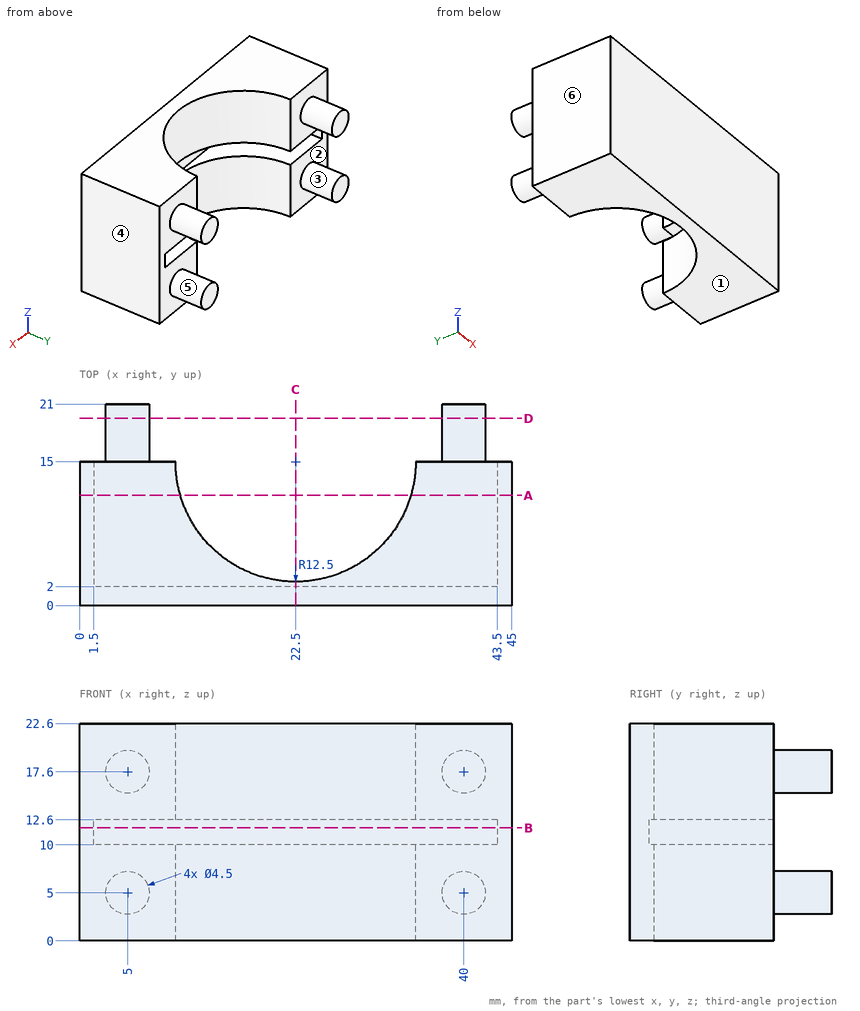
Job drawing, mm, ordinate dimensions from the low corner. One solid piece. A direction names the side the tool comes from. Round coordinates to 2 decimals unless told otherwise and drop trailing zeros. Write each loop counter-clockwise with the first axis right and the second up, starting at its lowest first coordinate (ties: lowest second). Pieces come first, ordered by that corner, then holes. Notation, with made-up numbers: (60, 65) -> (77, 65) arc R25 ccw to (77, 78) -> close; hole circle Ø5 at (31.5, 42.5). An arc over 180 degrees is marked (long way). Answer as a JSON object with one key per item and string values.
(1) Two-plate mould, pull along Z, no slides. Class the marked faces 1, 2, 3 and 4: +Z half, -Z half, draft (parallel to the pull), parting line (faces both ways), or undercut.
Reported:
{"face 1": "-Z half", "face 2": "undercut", "face 3": "undercut", "face 4": "draft"}
(2) Which spindle directions (+Z, -Z, +X, -X, +Y, -Y) get a long thin tool onto all of the face, cutting with end or side? Do the marked faces 5 and 6. Say none if no direction does.
Reported:
{"face 5": "+Y", "face 6": "+Z, -Z, -X, +Y, -Y"}
(3) Band-saw the part on A-A, the plane y = 11.5. List the corners of the cut face in (x, z), then the cut area to 3 significant figures.
Reported:
{"outline": "(0, 0) -> (10.5, 0) -> (10.5, 10) -> (1.5, 10) -> (1.5, 12.6) -> (10.5, 12.6) -> (10.5, 22.6) -> (0, 22.6) -> close; (34.5, 0) -> (45, 0) -> (45, 22.6) -> (34.5, 22.6) -> (34.5, 12.6) -> (43.5, 12.6) -> (43.5, 10) -> (34.5, 10) -> close", "area": "428 mm^2"}
(4) Band-saw the part on B-B, the plane z = 11.75. List the corners of the cut face in (x, y), then the cut area to 3 significant figures.
Reported:
{"outline": "(0, 0) -> (45, 0) -> (45, 15) -> (43.5, 15) -> (43.5, 2) -> (1.5, 2) -> (1.5, 15) -> (0, 15) -> close", "area": "129 mm^2"}
(5) Band-saw the part on D-D, the plane y = 19.5. List the corners of the cut face in (x, z), then the cut area to 3 significant figures.
Reported:
{"outline": "circle Ø4.5 at (5, 5); circle Ø4.5 at (5, 17.6); circle Ø4.5 at (40, 5); circle Ø4.5 at (40, 17.6)", "area": "63.6 mm^2"}
(6) Band-saw the part on C-C, the plane x = 22.5. List the corners of the cut face in (y, z).
Reported:
{"outline": "(0, 0) -> (2.5, 0) -> (2.5, 10) -> (2, 10) -> (2, 12.6) -> (2.5, 12.6) -> (2.5, 22.6) -> (0, 22.6) -> close"}
(7) Pin check, flat tips, straight feed: P1, Ø6, axis at x = 33.5, z = 10.5, coming from the +Y side; P2, Ø10, axis at x = 20, z = 20, coming from the +Y side. Stop position of each tip, or through.
Reported:
{"P1": "stops at y = 15", "P2": "stops at y = 5"}
(8) Probe probe 1 along X at (y, z) = (11, 12); probe 2 along Z at (x, y) = (33, 5); probe 3 along Y at (x, z) = (36.5, 2). List the from-to ranges inside material, lowest first. Write a range as [from, to].
Reported:
{"probe 1": "x = [0, 1.5], [43.5, 45]", "probe 2": "z = [0, 10], [12.6, 22.6]", "probe 3": "y = [0, 15]"}
